Could you check a few things on this model? Use its own coordinates, in mm. A direction names the side the tool comes from. Coordinates: 2 decimals unless noted, no trailing zeros. Write each loop counter-clockwise with the first axis right and the second up, starting at its lowest first coordinate (ties: lowest second). Pieces come first, ordered by that corner, then holes. Notation, with made-up numbers: (22.5, -26.5) - (78.5, -26.5) arc R27 cw to (78.5, -5.5) - close; hole circle Ø2 at (82, 37). An arc over 180 degrees is marked (long way). Answer as a JSON object with one key per item and string values. Group by question number.
1) If we section it at A-A (z = 38.1): Write out the boundary of the cut face in (x, y).
2) If we section it at C-C (z = 20): Write out the boundary of the cut face in (x, y), plus the area to 3 significant figures.
3) Will these pins go through, and if not, where does the flat tip stop? pin 1 Ø1 at (x, y) = (13, 261) entering from +Z; pin 2 Ø2 at (x, z) = (18.5, 19.5) entering from +Y; pin 3 Ø14 at (x, z) = (83, 3.5) entering from +Y.
4) On a 3-axis mill with a long thin cutter (end or side, diameter ignored), from which of +Z, -Z, +X, -X, +Y, -Y can I reach the whole of each face in a straight line? I mean faces 4 (the flat face through (50, 133.664, 31)), 5 (the flat face through (50, 140.014, 32)), 6 (the flat face through (79, 160.02, 6)). Say none if no direction works.
5) If we section it at D-D (y = 180.5): State how many separate pieces and enclosed holes the cut face has, plus the area to 3 significant figures.
6) We'd pull the mould along Z, two halves only. Please class faces 1 (the flat face through (101.6, 139, 24)), 2 (the flat face through (40, 184, 12.7)), 3 (the cylindrical face through (49.272, 136.883, 41.737)): released by +Z, released by -Z, zero draft, split by the parting line, or undercut.
7) Please list where these lines run through material, in increasing order: line 1 along X through (y, z) = (136.5, 38.1); line 2 along Z through (x, y) = (71.5, 202); line 3 along Y through (x, z) = (70, 31.5).
8) If we section it at B-B (y = 146): Write out the boundary of the cut face in (x, z).
```python
from build123d import *

# Parameters (mm, degrees)
SKETCH1_W           = 101.6
SKETCH1_H           = 152.4
BOSS_EXTRUDE1_DEPTH = 12.7
BOSS_EXTRUDE3_DEPTH = 12.7
FILLET1_R           = 2.54
FILLET2_R           = 5.08
CUT_EXTRUDE2_DEPTH  = 298.570512784
SKETCH8_W           = 101.6
SKETCH8_H           = 6.35
BOSS_EXTRUDE4_DEPTH = 50.8
SKETCH9_R           = 3.937
CUT_EXTRUDE3_DEPTH  = 184.802308472


with BuildPart() as part:
    # Sketch1 → Boss-Extrude1 (new body)
    with BuildSketch(Plane.XY):
        with Locations((50.8, 76.2)):
            Rectangle(SKETCH1_W, SKETCH1_H)
    extrude(amount=BOSS_EXTRUDE1_DEPTH)

    # Sketch2 → Boss-Extrude3 (add)
    with BuildSketch(Plane.XY):
        with BuildLine():
            add(Edge.make_bspline(
                [(0, 152.4), (39.790111277, 186.839065643), (12.30975625, 238.845497073), (0, 279.4)],
                knots=[0, 0, 0, 0, 1, 1, 1, 1], degree=3))
            add(Edge.make_bspline(
                [(0, 279.4), (51.286050257, 256.550041835), (87.836892382, 205.957944637), (101.6, 152.4)],
                knots=[0, 0, 0, 0, 1, 1, 1, 1], degree=3))
            Line((101.6, 152.4), (0, 152.4))
        make_face()
        with BuildLine():
            add(Edge.make_bspline(
                [(49.225838487, 233.315766274), (35.641228944, 236.267866949), (22.375615267, 231.937259722)],
                knots=[0, 0, 0, 1, 1, 1], degree=2))
            add(Edge.make_bspline(
                [(48.400350721, 207.535437601), (42.054170901, 227.566198031), (22.375615267, 231.937259722)],
                knots=[0, 0, 0, 1, 1, 1], degree=2))
            add(Edge.make_bspline(
                [(48.400350721, 207.535437601), (44.393568943, 220.734513873), (49.225838487, 233.315766274)],
                knots=[0, 0, 0, 1, 1, 1], degree=2))
        make_face(mode=Mode.SUBTRACT)
        with BuildLine():
            add(Edge.make_bspline(
                [(43.05348098, 206.08803494), (36.239789994, 218.91266054), (23.516066372, 224.861937296)],
                knots=[0, 0, 0, 1, 1, 1], degree=2))
            add(Edge.make_bspline(
                [(23.516066372, 224.861937296), (28.235295407, 215.21927262), (26.605728117, 204.582177714)],
                knots=[0, 0, 0, 1, 1, 1], degree=2))
            add(Edge.make_bspline(
                [(26.605728117, 204.582177714), (34.700432609, 206.792891754), (43.05348098, 206.08803494)],
                knots=[0, 0, 0, 1, 1, 1], degree=2))
        make_face(mode=Mode.SUBTRACT)
        with BuildLine():
            add(Edge.make_bspline(
                [(82.396089655, 183.81371778), (70.6713649, 174.663598784), (70.32777317, 160.02)],
                knots=[0, 0, 0, 1, 1, 1], degree=2))
            Line((70.32777317, 160.02), (87.546521436, 160.02))
            add(Edge.make_bspline(
                [(82.396089655, 183.81371778), (89.339550367, 172.773814043), (87.546521436, 160.02)],
                knots=[0, 0, 0, 1, 1, 1], degree=2))
        make_face(mode=Mode.SUBTRACT)
        with BuildLine():
            add(Edge.make_bspline(
                [(26.980466376, 183.81374211), (28.958775605, 170.837543608), (21.602944743, 160.02)],
                knots=[0, 0, 0, 1, 1, 1], degree=2))
            Line((21.602944743, 160.02), (40.676641776, 160.02))
            add(Edge.make_bspline(
                [(26.980466376, 183.81374211), (36.13847285, 173.175056715), (40.676641776, 160.02)],
                knots=[0, 0, 0, 1, 1, 1], degree=2))
        make_face(mode=Mode.SUBTRACT)
        with BuildLine():
            add(Edge.make_bspline(
                [(54.97708308, 160.02), (46.08347584, 181.54755316), (28.342136903, 196.529802482)],
                knots=[0, 0, 0, 1, 1, 1], degree=2))
            add(Edge.make_bspline(
                [(28.342136903, 196.529802482), (53.017815002, 201.732288521), (77.187204495, 194.363538628)],
                knots=[0, 0, 0, 1, 1, 1], degree=2))
            add(Edge.make_bspline(
                [(54.97708308, 160.02), (59.374728895, 181.400643158), (77.187204495, 194.363538628)],
                knots=[0, 0, 0, 1, 1, 1], degree=2))
        make_face(mode=Mode.SUBTRACT)
        with BuildLine():
            add(Edge.make_bspline(
                [(70.328259561, 206.277457578), (62.361576962, 208.669014941), (54.287141362, 207.109917469)],
                knots=[0, 0, 0, 1, 1, 1], degree=2))
            add(Edge.make_bspline(
                [(54.287141362, 207.109917469), (53.482096811, 217.391663167), (54.97708308, 227.557269012)],
                knots=[0, 0, 0, 1, 1, 1], degree=2))
            add(Edge.make_bspline(
                [(54.97708308, 227.557269012), (66.645859754, 219.852180834), (70.328259561, 206.277457578)],
                knots=[0, 0, 0, 1, 1, 1], degree=2))
        make_face(mode=Mode.SUBTRACT)
        with BuildLine():
            add(Edge.make_bspline(
                [(21.602944743, 238.323137826), (19.95197567, 252.974545225), (11.094737768, 264.601494061)],
                knots=[0, 0, 0, 1, 1, 1], degree=2))
            add(Edge.make_bspline(
                [(11.094737768, 264.601494061), (28.053835186, 259.295838115), (38.412267282, 244.949944056)],
                knots=[0, 0, 0, 1, 1, 1], degree=2))
            add(Edge.make_bspline(
                [(21.602944743, 238.323137826), (31.864782779, 237.284469605), (38.412267282, 244.949944056)],
                knots=[0, 0, 0, 1, 1, 1], degree=2))
        make_face(mode=Mode.SUBTRACT)
    extrude(amount=BOSS_EXTRUDE3_DEPTH)

    # Fillet1
    fillet1_edges = [part.edges().sort_by_distance(p)[0] for p in [
        (101.6, 152.4, 6.35),
        (0, 152.4, 6.35),
    ]]
    fillet(fillet1_edges, radius=FILLET1_R)

    # Fillet2
    fillet2_edges = [part.edges().sort_by_distance(p)[0] for p in [
        (0, 0, 6.35),
        (101.6, 0, 6.35),
    ]]
    fillet(fillet2_edges, radius=FILLET2_R)

    # Sketch5 → Cut-Extrude2 (cut, through all)
    with BuildSketch(Plane.XY.offset(12.7)):
        with BuildLine():
            Line((101.6, 133.663922723), (101.519048921, 133.663922723))
            Line((101.519048921, 133.663922723), (0, 133.663922723))
            Line((0, 133.663922723), (0, 5.08))
            ThreePointArc((0, 5.08), (1.487897552, 1.487897552), (5.08, 0))
            Line((5.08, 0), (96.52, 0))
            ThreePointArc((96.52, 0), (100.112102448, 1.487897552), (101.6, 5.08))
            Line((101.6, 5.08), (101.6, 133.663922723))
        make_face()
    extrude(amount=-CUT_EXTRUDE2_DEPTH, mode=Mode.SUBTRACT)

    # Sketch8 → Boss-Extrude4 (add)
    with BuildSketch(Plane.XY.offset(12.7)):
        with Locations((50.8, 136.838922723)):
            Rectangle(SKETCH8_W, SKETCH8_H)
    extrude(amount=BOSS_EXTRUDE4_DEPTH)

    # Sketch9 → Cut-Extrude3 (cut, through all)
    with BuildSketch(Plane(origin=(0, 140.013922723, 0), x_dir=(1, 0, 0), z_dir=(0, 1, 0))):
        with Locations(Location((50.77976223, -38.1, 0), (0, 0, 270))):
            Circle(SKETCH9_R)
    extrude(amount=-CUT_EXTRUDE3_DEPTH, mode=Mode.SUBTRACT)


solid = part.part
```
Here are the results:
{
 "1": {"outline": "(0, 133.66) - (46.84, 133.66) - (46.84, 140.01) - (0, 140.01) - close; (54.72, 133.66) - (101.6, 133.66) - (101.6, 140.01) - (54.72, 140.01) - close"},
 "2": {"outline": "(0, 133.66) - (101.6, 133.66) - (101.6, 140.01) - (0, 140.01) - close", "area": "645 mm²"},
 "3": {"pin 1": "stops at z = 12.7", "pin 2": "stops at y = 140.01", "pin 3": "stops at y = 211.57"},
 "4": {"face 4": "+Z, -Z, +X, -X, -Y", "face 5": "+Z, +X, -X, +Y", "face 6": "+Z, -Z"},
 "5": {"separate pieces": "4", "enclosed holes": "0", "area": "582 mm²"},
 "6": {"face 1": "zero draft", "face 2": "released by +Z", "face 3": "undercut"},
 "7": {"line 1": "x = 0 to 46.84, 54.72 to 101.6", "line 2": "z = 0 to 12.7", "line 3": "y = 133.66 to 140.01"},
 "8": {"outline": "(0, 0) - (101.6, 0) - (101.6, 12.7) - (0, 12.7) - close"}
}
